```python
from build123d import *

# Parameters (mm, degrees)
F0_W     = 13.1826
F0_H     = 6.985
F1_DEPTH = 13.2842
F2_R     = 3.175
F3_DEPTH = 7.9756


with BuildPart() as f1:
    # F0 (on Top) → F1 (new body)
    with BuildSketch(Plane.XY):
        Rectangle(F0_W, F0_H)
    extrude(amount=F1_DEPTH)

    # F2 (on face) → F3 (join)
    with BuildSketch(Plane.XY.offset(13.2842)):
        Circle(F2_R)
    extrude(amount=F3_DEPTH)

    # F5 (on offset) → F6 (revolve)
    with BuildSketch(Plane.XZ):
        with BuildLine():
            Line((-5.8194979442, 33.6655315498), (-1.3858759776, 21.2598))
            Line((-1.3858759776, 21.2598), (-0.4049631825, 21.2598))
            Line((-0.4049631825, 21.2598), (-3.8814046251, 32.6904004058))
            ThreePointArc((-3.8814046251, 32.6904004058), (-4.6416068333, 33.5930486447), (-5.8194979442, 33.6655315498))
        make_face()
    revolve(axis=Axis((-3.6026869609, 0, 27.4626657749), (0.3365385867, 0, -0.9416696765)))


solid = f1.part
```
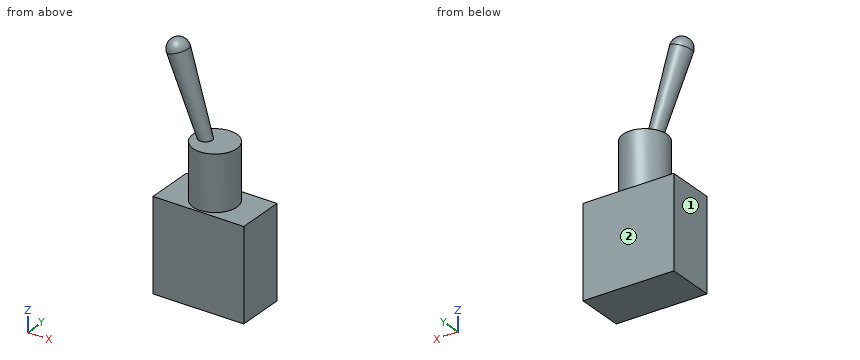
Geometry check sheet. Reference: the model listing, model coordinates, mm. Face numbers are marked on the shaded views. A direction names the side the tool comes from. Coordinates: 2 decimals unless noted, no trailing zeros. Loops run counter-clockwise (first coordinate to the right, second up) from the corner with the lowest first, then second, coordinate; pieces in that order, holes last.
Item 1: Access from +Z, -Z, +X, -X, +Y, -Y to the whole of each face (thin tool, end or side, straight path). Record for the marked faces 1 and 2.
Item 2: Go/stop test with flat-tipped pins: pin 1 Ø5 at (x, z) = (3, 19.5) entering from +Y; pin 2 Ø4 at (y, z) = (-0.5, 22) entering from -X; pin 3 Ø4 at (x, y) = (1, -2.5) entering from +Z. Record where each tip stops, or that it passes through.
Item 3: Sectioned sample at B-B, the plane y = 2. Record the boundary of the cut face in (x, z), then the cut area to 3 significant figures.
Item 4: Sectioned sample at C-C, the plane z = 4.5. Record the boundary of the cut face in (x, y), then the cut area to 3 significant figures.
Item 5: Thickness scan on line 1 (Z direction, x = -0.5, y = -2.5); line 2 (Z direction, x = 5, y = 1.25); line 3 (X direction, y = -2.25, z = 12). Record the ranges inside material, lowest first.
Item 6: Sectioned sample at D-D, the plane y = 0. Record the boundary of the cut face in (x, z) (1 decimal).
Check result:
1. face 1: -Z, -X, +Y, -Y
1. face 2: +Z, -Z, +X, -X, +Y
2. pin 1: stops at y = 3.14
2. pin 2: stops at x = -3.51
2. pin 3: stops at z = 21.26
3. outline: (-6.59, 0) - (6.59, 0) - (6.59, 13.28) - (2.47, 13.28) - (2.47, 21.26) - (-2.47, 21.26) - (-2.47, 13.28) - (-6.59, 13.28) - close
3. area: 214 mm2
4. outline: (-6.59, -3.49) - (6.59, -3.49) - (6.59, 3.49) - (-6.59, 3.49) - close
4. area: 92.1 mm2
5. line 1: z = 0 to 21.26
5. line 2: z = 0 to 13.28
5. line 3: x = -6.59 to 6.59
6. outline: (-6.7, 31.7) - (-2.4, 21.3) - (-3.2, 21.3) - (-3.2, 13.3) - (-6.6, 13.3) - (-6.6, 0) - (6.6, 0) - (6.6, 13.3) - (3.2, 13.3) - (3.2, 21.3) - (-0.4, 21.3) - (-3.9, 32.7) arc R1.5 ccw (long way) to start
